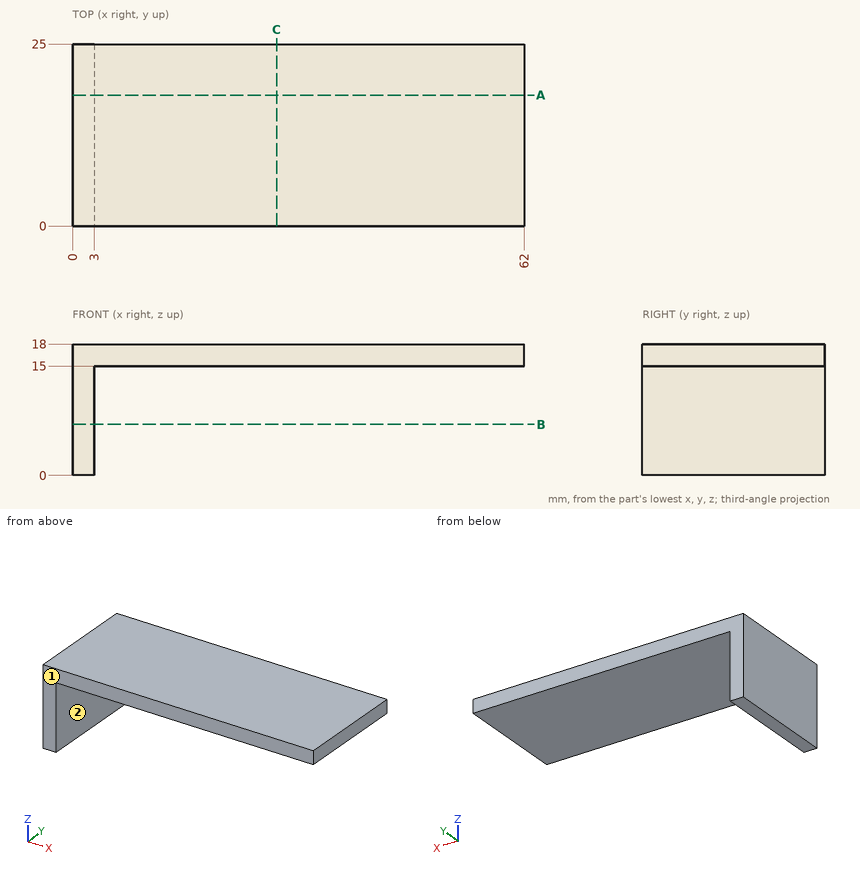
Input: dimensioned drawing with shaded views. Units: mm. Origin: part minimum x, y, z. A direction names the side the tool comes from. Round coordinates to 2 decimals unless told otherwise and drop trailing zeros. Loops run counter-clockwise (first coordinate to the right, second up) from the corner with the lowest first, then second, coordinate; pieces in that order, holes last. Notation, with made-up numbers: M 21,29.5 L 42,29.5 A13 cw 42,45.5 Z; hole C 79.5,65 d4. An arc over 180 degrees is marked long. Return JSON: item names as keys, results as strings. Group by question number.
1. Pin query (flat end, axial travel): pin 1 (10 mm diameter, centred on x = 28, y = 12.5, fed in from -Z); pin 2 (8 mm diameter, centred on y = 14, z = 10.5, fed in from +X). Return the tip coordinate at first contact, or that it passes through.
2. Material intervals for line 1 along Z through (x, y) = (56, 18.5); line 2 along X through (y, z) = (3.5, 14.5), sorted ascending. Write a range as from..to.
3. Section query B-B on z = 7. Output: boundary loops of the cut face in (x, y), and give its area (3 significant figures).
4. Reachability of the marked faces 1 and 2 from +Z, -Z, +X, -X, +Y, -Y: full face, straight path, thin tool, end or side. Return the list, or none.
5. Section query A-A on y = 18. Output: boundary loops of the cut face in (x, z), and give its area (3 significant figures).
6. Section query C-C on x = 28. Output: boundary loops of the cut face in (y, z), and give its area (3 significant figures).
Checks:
{
 "1": {"pin 1": "stops at z = 15", "pin 2": "stops at x = 3"},
 "2": {"line 1": "z = 15..18", "line 2": "x = 0..3"},
 "3": {"outline": "M 0,0 L 3,0 L 3,25 L 0,25 Z", "area": "75.0 mm²"},
 "4": {"face 1": "+Z, -Z, +X, -X, -Y", "face 2": "-Z, +X, +Y, -Y"},
 "5": {"outline": "M 0,0 L 3,0 L 3,15 L 62,15 L 62,18 L 0,18 Z", "area": "231 mm²"},
 "6": {"outline": "M 0,15 L 25,15 L 25,18 L 0,18 Z", "area": "75.0 mm²"}
}
